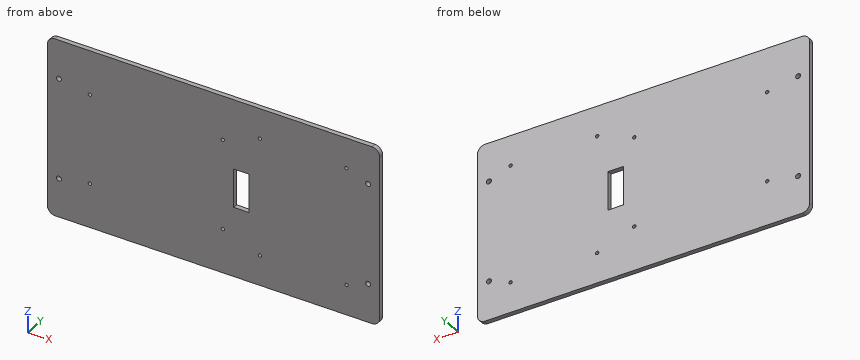
from build123d import *

# Parameters (mm, degrees)
SKETCH1_W           = 215
SKETCH1_H           = 115
SKETCH1_R           = 1.6
SKETCH1_R_2         = 1.1
SKETCH1_W_2         = 10
SKETCH1_H_2         = 25
BOSS_EXTRUDE1_DEPTH = 3
FILLET1_R           = 5


with BuildPart() as part:
    # Sketch1 → Boss-Extrude1 (new body)
    with BuildSketch(Plane(origin=(0, 0, 0), x_dir=(1, 0, 0), z_dir=(0, 1, 0))):
        Rectangle(SKETCH1_W, SKETCH1_H)
        with Locations(Location((100, -32.5, 0), (0, 0, 270))):
            Circle(SKETCH1_R, mode=Mode.SUBTRACT)
        with Locations(Location((-100, -32.5, 0), (0, 0, 90))):
            Circle(SKETCH1_R, mode=Mode.SUBTRACT)
        with Locations(Location((100, 32.5, 0), (0, 0, 90))):
            Circle(SKETCH1_R, mode=Mode.SUBTRACT)
        with Locations(Location((-100, 32.5, 0), (0, 0, 270))):
            Circle(SKETCH1_R, mode=Mode.SUBTRACT)
        with Locations(Location((-80, 29, 0), (0, 0, 270))):
            Circle(SKETCH1_R_2, mode=Mode.SUBTRACT)
        with Locations(Location((-80, -29, 0), (0, 0, 90))):
            Circle(SKETCH1_R_2, mode=Mode.SUBTRACT)
        with Locations(Location((30, 38, 0), (0, 0, 270))):
            Circle(SKETCH1_R_2, mode=Mode.SUBTRACT)
        with Locations(Location((86, 38, 0), (0, 0, 270))):
            Circle(SKETCH1_R_2, mode=Mode.SUBTRACT)
        with Locations(Location((86, -38, 0), (0, 0, 90))):
            Circle(SKETCH1_R_2, mode=Mode.SUBTRACT)
        with Locations(Location((30, -38, 0), (0, 0, 90))):
            Circle(SKETCH1_R_2, mode=Mode.SUBTRACT)
        with Locations(Location((6, 29, 0), (0, 0, 270))):
            Circle(SKETCH1_R_2, mode=Mode.SUBTRACT)
        with Locations(Location((6, -29, 0), (0, 0, 90))):
            Circle(SKETCH1_R_2, mode=Mode.SUBTRACT)
        with Locations((18, 0)):
            Rectangle(SKETCH1_W_2, SKETCH1_H_2, mode=Mode.SUBTRACT)
    extrude(amount=BOSS_EXTRUDE1_DEPTH)

    # Fillet1
    fillet1_edges = [part.edges().sort_by_distance(p)[0] for p in [
        (107.5, 1.5, 57.5),
        (-107.5, 1.5, 57.5),
        (-107.5, 1.5, -57.5),
        (107.5, 1.5, -57.5),
    ]]
    fillet(fillet1_edges, radius=FILLET1_R)


solid = part.part
Verification items for the finished model (mm, model axes). Round coordinates to 2 decimals unless told otherwise and drop trailing zeros. Loops run counter-clockwise (first coordinate to the right, second up) from the corner with the lowest first, then second, coordinate; pieces in that order, holes last. Notation, with made-up numbers: (19, 80.25) - (31, 80.25) arc R22 cw to (31, 86.25) - close; hole circle Ø9 at (80.25, -26). An arc over 180 degrees is marked (long way). Use a Markdown table: item, result. Add a question column.
1. Gauge pin test, flat ends, axial feed: pin 1 (3 mm diameter, centred on x = 100, z = 32.5, fed in from -Y); pin 2 (3 mm diameter, centred on x = 30, z = 38, fed in from +Y). Record the tip position at first contact, or that the pin passes through.
2. Section check A-A, the plane z = -3. Record the boundary of the cut face in (x, y), plus the area to 3 significant figures.
3. Section check B-B, the plane x = 17. Record the boundary of the cut face in (y, z), plus the area to 3 significant figures.
4. Thickness scan on probe 1 along X at (y, z) = (1.6, -29); probe 2 along X at (y, z) = (0.75, 32.5); probe 3 along Z at (x, y) = (-100, 1.35). Record the ranges inside material, lowest first. Write a range as [from, to].
Checks:
| question | item | result |
|---|---|---|
| 1 | pin 1 | passes through |
| 1 | pin 2 | stops at y = 3 |
| 2 | outline | (-107.5, 0) - (13, 0) - (13, 3) - (-107.5, 3) - close; (23, 0) - (107.5, 0) - (107.5, 3) - (23, 3) - close |
| 2 | area | 615 mm^2 |
| 3 | outline | (0, -57.5) - (3, -57.5) - (3, -12.5) - (0, -12.5) - close; (0, 12.5) - (3, 12.5) - (3, 57.5) - (0, 57.5) - close |
| 3 | area | 270 mm^2 |
| 4 | probe 1 | x = [-107.5, -81.1], [-78.9, 4.9], [7.1, 107.5] |
| 4 | probe 2 | x = [-107.5, -101.6], [-98.4, 98.4], [101.6, 107.5] |
| 4 | probe 3 | z = [-57.5, -34.1], [-30.9, 30.9], [34.1, 57.5] |
